Input: part model. Units: mm. Frame: model coordinates. A direction names the side the tool comes from. Coordinates: 2 decimals unless noted, no trailing zeros. Write each loop counter-clockwise with the first axis right and the second up, starting at its lowest first coordinate (ties: lowest second). Pieces come first, ordered by that corner, then holes.
from build123d import *

# Parameters (mm, degrees)
F0_W     = 323.85
F0_H     = 209.55
F1_DEPTH = 171.45
F2_R     = 79.375
F3_DEPTH = 171.451
F4_W     = 69.421232
F4_H     = 41.941766
F5_DEPTH = 76.2


with BuildPart() as f1:
    # F0 (on Top) → F1 (new body)
    with BuildSketch(Plane.XY):
        with Locations((161.925, 104.775)):
            Rectangle(F0_W, F0_H)
    extrude(amount=F1_DEPTH)

    # F2 (on face) → F3 (cut, through all)
    with BuildSketch(Plane.XY.offset(171.45)):
        with Locations((92.075, 104.775)):
            Circle(F2_R)
    extrude(amount=-F3_DEPTH, mode=Mode.SUBTRACT)

    # F4 (on face) → F5 (cut)
    with BuildSketch(Plane.XZ):
        with Locations((269.471973, 46.484394)):
            Rectangle(F4_W, F4_H)
    extrude(amount=-F5_DEPTH, mode=Mode.SUBTRACT)


solid = f1.part
Item 1: Section query B-B, the plane x = 267.5. Return loops of the section in (y, z), then the cut area to 3 significant figures.
Item 2: Pull-direction query (Z, two-part tool) for faces 1 (the face through (234.761, 38, 46)), 2 (the face through (196, 106, 0)), 3 (the face through (0, 103, 85)); classes: released by +Z, released by -Z, zero draft, split by the parting line, or undercut.
Item 3: Access query for faces 4 (the face through (323.85, 103, 85)), 5 (the face through (269, 38, 67.455)). Directions: +Z, -Z, +X, -X, +Y, -Y. A direction counts if a zero-diameter tool reaches every point of the face in a straight line with its end or side. Return the directions, or none.
Item 4: Pin query (flat end, axial travel): pin 1 Ø3 at (x, z) = (238.5, 70) entering from -Y; pin 2 Ø21 at (x, z) = (255, 48.5) entering from -Y. Return the tip coordinate at first contact, or that it passes through.
Item 5: Section query A-A, the plane y = 110. Return loops of the section in (x, z), then the cut area to 3 significant figures.
Item 6: Material intervals for line 1 (X direction, y = 13, z = 67); line 2 (X direction, y = 105, z = 134.5); line 3 (X direction, y = 37.5, z = 63), sorted ascending.
Item 7: Section query C-C, the plane z = 45.5. Return loops of the section in (x, y) (3 decimals), then the cut area to 3 significant figures.
Item 8: Section query D-D, the plane x = 118.5. Return loops of the section in (y, z), then the cut area to 3 significant figures.
The answers:
1. outline: (0, 0) - (209.55, 0) - (209.55, 171.45) - (0, 171.45) - (0, 67.46) - (76.2, 67.46) - (76.2, 25.51) - (0, 25.51) - close
1. area: 32,700 mm2
2. face 1: undercut
2. face 2: released by -Z
2. face 3: zero draft
3. face 4: +Z, -Z, +X, +Y, -Y
3. face 5: -Y
4. pin 1: stops at y = 0
4. pin 2: stops at y = 76.2
5. outline: (0, 0) - (12.87, 0) - (12.87, 171.45) - (0, 171.45) - close; (171.28, 0) - (323.85, 0) - (323.85, 171.45) - (171.28, 171.45) - close
5. area: 28,400 mm2
6. line 1: x = 0 to 234.76, 304.18 to 323.85
6. line 2: x = 0 to 12.7, 171.45 to 323.85
6. line 3: x = 0 to 49.95, 134.2 to 234.76, 304.18 to 323.85
7. outline: (0, 0) - (234.761, 0) - (234.761, 76.2) - (304.183, 76.2) - (304.183, 0) - (323.85, 0) - (323.85, 209.55) - (0, 209.55) - close; hole circle Ø158.75 at (92.075, 104.775)
7. area: 42,800 mm2
8. outline: (0, 0) - (29.93, 0) - (29.93, 171.45) - (0, 171.45) - close; (179.62, 0) - (209.55, 0) - (209.55, 171.45) - (179.62, 171.45) - close
8. area: 10,300 mm2
